Check sheet for the modelled part. Datum: model origin and axes. Units: mm. Face numbers are marked on the shaded views. A direction names the side the tool comes from. Give positions to 0.01 mm unless a question says otherwise; leave off trailing zeros. Order: outer loops, then holes, each group sorted by start corner. A loop starts at its lowest first (then second) coordinate and runs counter-clockwise, first axis right, second up. Notation, with made-up numbers: M 14.25,-20 L 20.25,-20 A20 cw 20.25,1 Z; hole C -21.5,86 d2. An arc over 180 degrees is marked long. Answer in a Markdown table with one row per item. Add a question column.
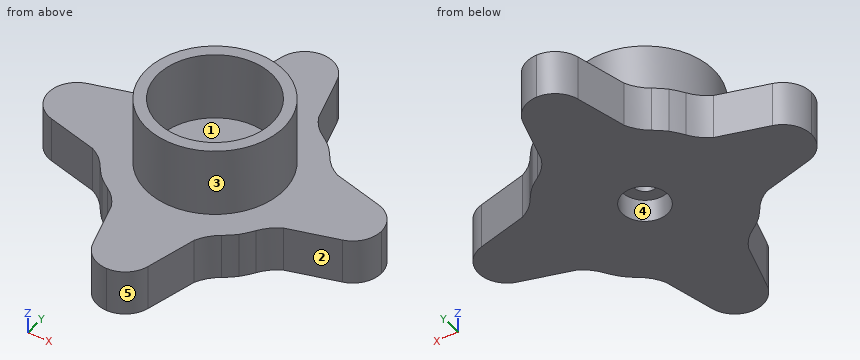
from build123d import *

# Parameters (mm, degrees)
BOSS_EXTRUDE1_DEPTH = 2
SKETCH2_R           = 3
SKETCH2_R_2         = 2.5
BOSS_EXTRUDE2_DEPTH = 3
SKETCH3_R           = 1
CUT_EXTRUDE1_DEPTH  = 1
SKETCH4_R           = 0.5
CUT_EXTRUDE2_DEPTH  = 12.407234547


with BuildPart() as part:
    # Sketch1 → Boss-Extrude1 (new body)
    with BuildSketch(Plane.XY):
        with BuildLine():
            Line((-1.2, 6.33), (-1.8, 4.16))
            ThreePointArc((-1.8, 4.16), (-2.089343599, 3.728660349), (-2.48, 3.386372183))
            ThreePointArc((-2.48, 3.386372183), (-2.740944688, 3.196252087), (-2.985706385, 2.985706385))
            ThreePointArc((-2.985706385, 2.985706385), (-3.196252087, 2.740944688), (-3.386372183, 2.48))
            ThreePointArc((-3.386372183, 2.48), (-3.728660349, 2.089343599), (-4.16, 1.8))
            Line((-4.16, 1.8), (-6.33, 1.2))
            ThreePointArc((-6.33, 1.2), (-6.992020752, 0.754882576), (-7.25, 0))
            ThreePointArc((-7.25, 0), (-6.992020752, -0.754882576), (-6.33, -1.2))
            Line((-6.33, -1.2), (-4.16, -1.8))
            ThreePointArc((-4.16, -1.8), (-3.728660349, -2.089343599), (-3.386372183, -2.48))
            ThreePointArc((-3.386372183, -2.48), (-3.196252087, -2.740944688), (-2.985706385, -2.985706385))
            ThreePointArc((-2.985706385, -2.985706385), (-2.740944688, -3.196252087), (-2.48, -3.386372183))
            ThreePointArc((-2.48, -3.386372183), (-2.089343599, -3.728660349), (-1.8, -4.16))
            Line((-1.8, -4.16), (-1.2, -6.33))
            ThreePointArc((-1.2, -6.33), (-0.754882576, -6.992020752), (0, -7.25))
            ThreePointArc((0, -7.25), (0.754882576, -6.992020752), (1.2, -6.33))
            Line((1.2, -6.33), (1.8, -4.16))
            ThreePointArc((1.8, -4.16), (2.089343599, -3.728660349), (2.48, -3.386372183))
            ThreePointArc((2.48, -3.386372183), (2.740944688, -3.196252087), (2.985706385, -2.985706385))
            ThreePointArc((2.985706385, -2.985706385), (3.196252087, -2.740944688), (3.386372183, -2.48))
            ThreePointArc((3.386372183, -2.48), (3.728660349, -2.089343599), (4.16, -1.8))
            Line((4.16, -1.8), (6.33, -1.2))
            ThreePointArc((6.33, -1.2), (6.992020752, -0.754882576), (7.25, 0))
            ThreePointArc((7.25, 0), (6.992020752, 0.754882576), (6.33, 1.2))
            Line((6.33, 1.2), (4.16, 1.8))
            ThreePointArc((4.16, 1.8), (3.728660349, 2.089343599), (3.386372183, 2.48))
            ThreePointArc((3.386372183, 2.48), (3.196252087, 2.740944688), (2.985706385, 2.985706385))
            ThreePointArc((2.985706385, 2.985706385), (2.740944688, 3.196252087), (2.48, 3.386372183))
            ThreePointArc((2.48, 3.386372183), (2.089343599, 3.728660349), (1.8, 4.16))
            Line((1.8, 4.16), (1.2, 6.33))
            ThreePointArc((1.2, 6.33), (0.754882576, 6.992020752), (0, 7.25))
            ThreePointArc((0, 7.25), (-0.754882576, 6.992020752), (-1.2, 6.33))
        make_face()
    extrude(amount=BOSS_EXTRUDE1_DEPTH)

    # Sketch2 → Boss-Extrude2 (add)
    with BuildSketch(Plane.XY.offset(2)):
        with Locations(Location((0, 0, 0), (0, 0, 180))):
            Circle(SKETCH2_R)
        Circle(SKETCH2_R_2, mode=Mode.SUBTRACT)
    extrude(amount=BOSS_EXTRUDE2_DEPTH)

    # Sketch3 → Cut-Extrude1 (cut)
    with BuildSketch(Plane(origin=(0, 0, 0), x_dir=(-1, 0, 0), z_dir=(0, 0, -1))):
        Circle(SKETCH3_R)
    extrude(amount=-CUT_EXTRUDE1_DEPTH, mode=Mode.SUBTRACT)

    # Sketch4 → Cut-Extrude2 (cut, through all)
    with BuildSketch(Plane.XY):
        with Locations(Location((0, 0, 0), (0, 0, 180))):
            Circle(SKETCH4_R)
    extrude(amount=CUT_EXTRUDE2_DEPTH, mode=Mode.SUBTRACT)


solid = part.part
Q1. Go/stop test with flat-tipped pins: pin 1 (3 mm diameter, centred on x = 0, y = 0, fed in from -Z); pin 2 (2.5 mm diameter, centred on x = 1, y = 0.5, fed in from +Z); pin 3 (1 mm diameter, centred on y = -4, z = 1.5, fed in from +X); pin 4 (1.5 mm diameter, centred on y = -3, z = 3.5, fed in from -X). Record where each tip stops, or that it passes through.
Q2. Thickness scan on probe 1 along Y at (x, z) = (0, 3.5); probe 2 along Z at (x, y) = (1, -4); probe 3 along Y at (x, z) = (-2.75, 4.45). Record the ranges inside material, lowest first.
Q3. Cross-section at D-D (y = 1.5). Record the boundary of the cut face in (x, z) (3 decimals).
Q4. Cross-section at B-B (y = -0.25). Record the boundary of the cut face in (x, z).
Q5. Tool access check on the marked faces 1 and 2. Record the directions out of +Z, -Z, +X, -X, +Y, -Y that give a thin tool (end or side, any length) a straight path to the whole face; none if there is none.
Q6. Draft check along Y on the marked faces 3, 4 and 5. Enter one of: pulls with the +Y half, pulls with the -Y half, needs draft (parallel to the pull), parting line crosses it, or undercut.
Values follow:
| question | item | result |
|---|---|---|
| 1 | pin 1 | z = 0 |
| 1 | pin 2 | z = 2 |
| 1 | pin 3 | x = 2.33 |
| 1 | pin 4 | x = -1.98 |
| 2 | probe 1 | -3 to -2.5, 2.5 to 3 |
| 2 | probe 2 | 0 to 2 |
| 2 | probe 3 | -1.2 to 1.2 |
| 3 | outline | M -5.245,0 L 5.245,0 L 5.245,2 L 2.598,2 L 2.598,5 L 2,5 L 2,2 L -2,2 L -2,5 L -2.598,5 L -2.598,2 L -5.245,2 Z |
| 4 | outline | M -7.22,0 L -0.97,0 L -0.97,1 L -0.43,1 L -0.43,2 L -2.49,2 L -2.49,5 L -2.99,5 L -2.99,2 L -7.22,2 Z; M 0.43,1 L 0.97,1 L 0.97,0 L 7.22,0 L 7.22,2 L 2.99,2 L 2.99,5 L 2.49,5 L 2.49,2 L 0.43,2 Z |
| 5 | face 1 | +Z |
| 5 | face 2 | +Z, -Z, +X, -Y |
| 6 | face 3 | parting line crosses it |
| 6 | face 4 | undercut |
| 6 | face 5 | pulls with the -Y half |
